```python
from build123d import *

# Parameters (mm, degrees)
SKETCH1_W             = 80
SKETCH1_H             = 225
BOSS_EXTRUDE1_DEPTH   = 10
CUT_EXTRUDE1_REACH    = 121.818
SKETCH2_R             = 6
M8_CLEARANCE_HOLE1_D  = 8.4
F_8_0MM_DOWEL_HOLE1_D = 8
CUT_EXTRUDE3_REACH    = 121.818
SKETCH10_R            = 7


with BuildPart() as part:
    # Sketch1 → Boss-Extrude1 (new body)
    with BuildSketch(Plane(origin=(0, 0, 0), x_dir=(1, 0, 0), z_dir=(0, 1, 0))):
        Rectangle(SKETCH1_W, SKETCH1_H)
    extrude(amount=-BOSS_EXTRUDE1_DEPTH)

    # Sketch2 → Cut-Extrude1 (cut, up to next)
    with BuildSketch(Plane(origin=(0, 0, 0), x_dir=(1, 0, 0), z_dir=(0, 1, 0)), mode=Mode.PRIVATE) as cut_extrude1_sk1:
        with Locations(Location((0, 77.5, 0), (0, 0, 270))):
            Circle(SKETCH2_R)
    cut_extrude1_tool1 = extrude(cut_extrude1_sk1.sketch, amount=-CUT_EXTRUDE1_REACH, mode=Mode.PRIVATE) & part.part
    # Sketch2 → Cut-Extrude1 (cut, up to next)
    with BuildSketch(Plane(origin=(0, 0, 0), x_dir=(1, 0, 0), z_dir=(0, 1, 0)), mode=Mode.PRIVATE) as cut_extrude1_sk2:
        with Locations(Location((30, 4, 0), (0, 0, 270))):
            Circle(SKETCH2_R)
    cut_extrude1_tool2 = extrude(cut_extrude1_sk2.sketch, amount=-CUT_EXTRUDE1_REACH, mode=Mode.PRIVATE) & part.part
    # Sketch2 → Cut-Extrude1 (cut, up to next)
    with BuildSketch(Plane(origin=(0, 0, 0), x_dir=(1, 0, 0), z_dir=(0, 1, 0)), mode=Mode.PRIVATE) as cut_extrude1_sk3:
        with Locations(Location((-30, 4, 0), (0, 0, 270))):
            Circle(SKETCH2_R)
    cut_extrude1_tool3 = extrude(cut_extrude1_sk3.sketch, amount=-CUT_EXTRUDE1_REACH, mode=Mode.PRIVATE) & part.part
    # Sketch2 → Cut-Extrude1 (cut, up to next)
    with BuildSketch(Plane(origin=(0, 0, 0), x_dir=(1, 0, 0), z_dir=(0, 1, 0)), mode=Mode.PRIVATE) as cut_extrude1_sk4:
        with Locations(Location((0, -77.5, 0), (0, 0, 270))):
            Circle(SKETCH2_R)
    cut_extrude1_tool4 = extrude(cut_extrude1_sk4.sketch, amount=-CUT_EXTRUDE1_REACH, mode=Mode.PRIVATE) & part.part
    add(cut_extrude1_tool1.solids().sort_by_distance((0, 0, -77.5))[0], mode=Mode.SUBTRACT)
    add(cut_extrude1_tool2.solids().sort_by_distance((30, 0, -4))[0], mode=Mode.SUBTRACT)
    add(cut_extrude1_tool3.solids().sort_by_distance((-30, 0, -4))[0], mode=Mode.SUBTRACT)
    add(cut_extrude1_tool4.solids().sort_by_distance((0, 0, 77.5))[0], mode=Mode.SUBTRACT)

    # M8 Clearance Hole1 (through all)
    with Locations(Plane(origin=(0, 0, 0), x_dir=(1, 0, 0), z_dir=(0, 1, 0))):
        with Locations((-25, 97.5), (25, 97.5), (25, -97.5), (-25, -97.5)):
            Hole(M8_CLEARANCE_HOLE1_D / 2)

    # Ø8.0mm Dowel Hole1 (through all)
    with Locations(Plane(origin=(0, 0, 0), x_dir=(1, 0, 0), z_dir=(0, 1, 0))):
        with Locations((25, 81.975), (-25, -82)):
            Hole(F_8_0MM_DOWEL_HOLE1_D / 2)

    # Sketch10 → Cut-Extrude3 (cut, up to next)
    with BuildSketch(Plane(origin=(0, 0, 0), x_dir=(1, 0, 0), z_dir=(0, 1, 0)), mode=Mode.PRIVATE) as cut_extrude3_sk1:
        with Locations(Location((0, 10.23, 0), (0, 0, 270))):
            Circle(SKETCH10_R)
    cut_extrude3_tool1 = extrude(cut_extrude3_sk1.sketch, amount=-CUT_EXTRUDE3_REACH, mode=Mode.PRIVATE) & part.part
    add(cut_extrude3_tool1.solids().sort_by_distance((0, 0, -10.23))[0], mode=Mode.SUBTRACT)


solid = part.part
```
Read the model definition and answer for the solid it produces. Units are mm, in the model's axes. Give positions to 0.01 mm unless a question says otherwise; leave off trailing zeros. Write each loop counter-clockwise with the first axis right and the second up, starting at its lowest first coordinate (ties: lowest second). Pieces come first, ordered by that corner, then holes. Notation, with made-up numbers: M 42,1 L 93,1 A28 ccw 93,19 Z; hole C -36.5,30 d8. An arc over 180 degrees is marked long. Put each result on its own line as item: value. Start each with the question number.
1. The part is cut by section B-B, the plane y = -7.5. Give the number of separate pieces and of enclosed holes in the cut face, and give its area (3 significant figures).
2. For a pull along X with two mould halves and no side action, classify faces 1 (the flat face through (-40, -5, 2)), 2 (the flat face through (-1, -10, -2)), 3 (the cylindrical face through (-35.857, -4.93, -5.301)) as released by +X, released by -X, zero draft, split by the parting line, or undercut.
3. The part is cut by section C-C, the plane x = -2. Give the vertices of the cut face in (y, z), and give its area (3 significant figures).
4. Consider line 1 along X through (y, z) = (-2.25, -97.5); line 2 along X through (y, z) = (-6.75, 77.5); line 3 along Z through (x, y) = (-25, -7.25). Determine where each line is inside the solid, lowest interval first.
5. The part is cut by section D-D, the plane z = -12.5. Give the vertices of the cut face in (x, y), and give its area (3 significant figures).
6. The part is cut by section A-A, the plane z = -97.5. Give the vertices of the cut face in (x, y), and give its area (3 significant figures).
Final values:
1. separate pieces: 1
1. enclosed holes: 11
1. area: 17,100 mm²
2. face 1: released by -X
2. face 2: zero draft
2. face 3: undercut
3. outline: M -10,-112.5 L 0,-112.5 L 0,-83.16 L -10,-83.16 Z; M -10,-71.84 L 0,-71.84 L 0,-16.94 L -10,-16.94 Z; M -10,-3.52 L 0,-3.52 L 0,71.84 L -10,71.84 Z; M -10,83.16 L 0,83.16 L 0,112.5 L -10,112.5 Z
3. area: 1,890 mm²
4. line 1: x = -40 to -29.2, -20.8 to 20.8, 29.2 to 40
4. line 2: x = -40 to -6, 6 to 40
4. line 3: z = -112.5 to -101.7, -93.3 to -7.32, -0.68 to 78, 86 to 93.3, 101.7 to 112.5
5. outline: M -40,-10 L -6.62,-10 L -6.62,0 L -40,0 Z; M 6.62,-10 L 40,-10 L 40,0 L 6.62,0 Z
5. area: 668 mm²
6. outline: M -40,-10 L -29.2,-10 L -29.2,0 L -40,0 Z; M -20.8,-10 L 20.8,-10 L 20.8,0 L -20.8,0 Z; M 29.2,-10 L 40,-10 L 40,0 L 29.2,0 Z
6. area: 632 mm²
